```python
from build123d import *

# Parameters (mm, degrees)
SKETCH_W        = 9.2
SKETCH_H        = 9.2
PAD_DEPTH       = 13
SKETCH002_W     = 6
SKETCH002_H     = 12
PAD001_DEPTH    = 1
SKETCH008_R     = 3
POCKET_DEPTH    = 2
SKETCH004_W     = 4.6
SKETCH004_H     = 9.2
POCKET001_DEPTH = 7.5
SKETCH009_R     = 0.5
POCKET002_DEPTH = 14.001
FILLET_R        = 1.2


with BuildPart() as part:
    # Sketch → Pad (new body)
    with BuildSketch(Plane.XY):
        Rectangle(SKETCH_W, SKETCH_H)
    extrude(amount=PAD_DEPTH)

    # Sketch002 → Pad001 (join)
    with BuildSketch(Plane(origin=(0, 0, 0), x_dir=(1, 0, 0), z_dir=(0, 0, -1))):
        with Locations((-3, 0)):
            Rectangle(SKETCH002_W, SKETCH002_H)
    extrude(amount=PAD001_DEPTH)

    # Sketch008 (on Face12 of Pad001) → Pocket (cut)
    with BuildSketch(Plane(origin=(0, 0, -1), x_dir=(1, 0, 0), z_dir=(0, 0, -1))):
        Circle(SKETCH008_R)
    extrude(amount=-POCKET_DEPTH, mode=Mode.SUBTRACT)

    # Sketch004 → Pocket001 (cut)
    with BuildSketch(Plane(origin=(0, 0, -2), x_dir=(1, 0, 0), z_dir=(0, 0, -1))):
        with Locations((2.3, 0)):
            Rectangle(SKETCH004_W, SKETCH004_H)
    extrude(amount=-POCKET001_DEPTH, mode=Mode.SUBTRACT)

    # Sketch009 (on Face6 of Pocket001) → Pocket002 (cut, through all)
    with BuildSketch(Plane.XY.offset(13)):
        Circle(SKETCH009_R)
    extrude(amount=-POCKET002_DEPTH, mode=Mode.SUBTRACT)

    # Fillet
    fillet_edges = [part.edges().sort_by_distance(p)[0] for p in [
        (-4.6, -4.6, 6.5),
        (0, -4.6, 13),
        (-4.6, 0, 13),
        (-4.6, 4.6, 6.5),
        (0, 4.6, 13),
        (4.6, 0, 13),
        (4.6, 4.6, 9.25),
        (4.6, -4.6, 9.25),
    ]]
    fillet(fillet_edges, radius=FILLET_R)


solid = part.part
```
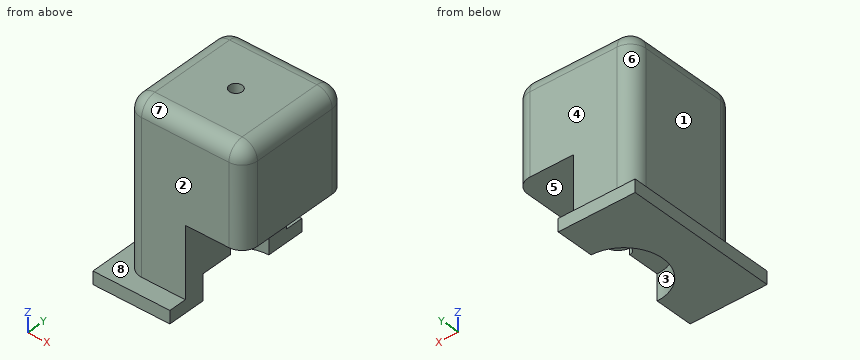
The listing builds one solid part. Answer for the finished solid, in the listing's coordinates (mm). Face numbers are marked on the shaded views. A direction names the side the tool comes from. Give positions to 0.01 mm unless a question says otherwise; leave off trailing zeros. Write each loop counter-clockwise with the first axis right and the second up, starting at its lowest first coordinate (ties: lowest second). Pieces come first, ordered by that corner, then holes. Notation, with made-up numbers: (41.5, 58.5) -> (58.5, 58.5) arc R21 ccw to (58.5, 68.5) -> close; hole circle Ø5 at (21.25, 24.5). An arc over 180 degrees is marked (long way). Use one line per item in the form item = value.
1) Section D-D on z = 0.75 is taken. Write down the section's boundary in (x, y), plus the area to 3 significant figures.
Result:
outline = (-4.6, -3.4) arc R1.2 ccw to (-3.4, -4.6) -> (0, -4.6) -> (0, -3) arc R3 cw to (0, 3) -> (0, 4.6) -> (-3.4, 4.6) arc R1.2 ccw to (-4.6, 3.4) -> close
area = 27.6 mm²
2) Section C-C on y = -2.75 is taken. Write down the section's boundary in (x, z).
Result:
outline = (-6, -1) -> (-1.2, -1) -> (-1.2, 1) -> (0, 1) -> (0, 5.5) -> (4.6, 5.5) -> (4.6, 11.8) arc R1.2 ccw to (3.4, 13) -> (-3.4, 13) arc R1.2 ccw to (-4.6, 11.8) -> (-4.6, 0) -> (-6, 0) -> close
3) For a pull along Y with two mould halves and no side action, classify the marked faces 1, 2 and 3 as +Y half, -Y half, draft (parallel to the pull), parting line (faces both ways), or undercut.
Result:
face_1 = draft
face_2 = -Y half
face_3 = undercut
4) Each of these flat-tipped pins is pushed along its axis until it touches: P1, Ø3.5, axis at y = 0.5, z = 4.5, coming from the -X side; P2, Ø1.6, axis at y = -4.5, z = 2.5, coming from the +X side; P3, Ø3.5, axis at x = 1, z = 5, coming from the +Y side. Where does it stop, or does it pass through?
Result:
P1 = -4.6
P2 = 0
P3 = 4.6
5) A tool of negligible diameter and unlimited length cuts with its end or side. For the marked faces 4, 5, 6, 7 and 8, from which of +Z, -Z, +X, -X, +Y, -Y can it reach the whole face along a straight path? Write none if from no direction.
Result:
face_4 = +Z, +X, -X, +Y
face_5 = -Z, +X, +Y, -Y
face_6 = +Z, -X, +Y
face_7 = +Z, +X, -X, -Y
face_8 = +Z, -X
6) Straight lines are drawn through the part: probe 1 along Y at (x, z) = (0, 10); probe 2 along Z at (x, y) = (-5, 4.25); probe 3 along X at (y, z) = (1.25, 4.5). For each, find the intervals that lie inside material, in ascending order.
Result:
probe_1 = -4.6 to -0.5, 0.5 to 4.6
probe_2 = -1 to 0
probe_3 = -4.6 to 0
7) Section B-B on z = 3 is taken. Write down the section's boundary in (x, y), plus the area to 3 significant figures.
Result:
outline = (-4.6, -3.4) arc R1.2 ccw to (-3.4, -4.6) -> (0, -4.6) -> (0, -0.5) arc R0.5 cw to (0, 0.5) -> (0, 4.6) -> (-3.4, 4.6) arc R1.2 ccw to (-4.6, 3.4) -> close
area = 41.3 mm²
8) Section A-A on y = 0 is taken. Write down the section's boundary in (x, z), plus the area to 3 significant figures.
Result:
outline = (-6, -1) -> (-3, -1) -> (-3, 1) -> (-0.5, 1) -> (-0.5, 13) -> (-3.4, 13) arc R1.2 ccw to (-4.6, 11.8) -> (-4.6, 0) -> (-6, 0) -> close; (0.5, 5.5) -> (4.6, 5.5) -> (4.6, 11.8) arc R1.2 ccw to (3.4, 13) -> (0.5, 13) -> close
area = 83.9 mm²
